```python
from build123d import *

# Parameters (mm, degrees)
SKETCH_W     = 210
SKETCH_H     = 82
SKETCH_R     = 1.65
PAD_DEPTH    = 1.5
POCKET_DEPTH = 1.501


with BuildPart() as part:
    # Sketch → Pad (new body)
    with BuildSketch(Plane.XZ):
        Rectangle(SKETCH_W, SKETCH_H)
        with Locations((100, 30)):
            Circle(SKETCH_R, mode=Mode.SUBTRACT)
        with Locations((100, 10)):
            Circle(SKETCH_R, mode=Mode.SUBTRACT)
        with Locations((100, -30)):
            Circle(SKETCH_R, mode=Mode.SUBTRACT)
        with Locations((100, -10)):
            Circle(SKETCH_R, mode=Mode.SUBTRACT)
        with Locations((-100, 30)):
            Circle(SKETCH_R, mode=Mode.SUBTRACT)
        with Locations((-100, 10)):
            Circle(SKETCH_R, mode=Mode.SUBTRACT)
        with Locations((-100, -30)):
            Circle(SKETCH_R, mode=Mode.SUBTRACT)
        with Locations((-100, -10)):
            Circle(SKETCH_R, mode=Mode.SUBTRACT)
    extrude(amount=PAD_DEPTH)

    # Sketch002 → Pocket (cut, through all)
    with BuildSketch(Plane.XZ.offset(1.5)):
        with BuildLine():
            ThreePointArc((-82.5, 12.5), (-95, 0), (-82.5, -12.5))
            Line((-82.5, -12.5), (82.5, -12.5))
            ThreePointArc((82.5, -12.5), (95, 0), (82.5, 12.5))
            Line((-82.5, 12.5), (82.5, 12.5))
        make_face()
    extrude(amount=-POCKET_DEPTH, mode=Mode.SUBTRACT)


solid = part.part
```
The model under review builds one solid part; all positions refer to its coordinate system, in mm. Coordinates: 2 decimals unless noted, no trailing zeros. Order: outer loops, then holes, each group sorted by start corner. A loop starts at its lowest first (then second) coordinate and runs counter-clockwise, first axis right, second up. Notation, with made-up numbers: M 67,38 L 124,38 A17 ccw 124,46 Z; hole C 82,22.5 d11. An arc over 180 degrees is marked long. One line per question, with ' | ' between items.
(1) The part is to be moulded in two halves that separate along X. For faces 1 (the face through (95, -1, 0)), 2 (the face through (-1, 0, 19)), 3 (the face through (-95, -1, 0)), say which applies: +X half, -X half, draft (parallel to the pull), parting line (faces both ways), or undercut.
Geometry results:
face 1: undercut | face 2: draft | face 3: undercut
(2) Add section C-C, the plane y = -1.15. State how many separate pieces and enclosed holes the cut face has, then the cut area to 3 significant figures.
Geometry results:
separate pieces: 1 | enclosed holes: 9 | area: 12,500 mm²
(3) Add section B-B, the plane z = 5. Write out the cut boundary in (x, y).
Geometry results:
outline: M -105,-1.5 L -93.96,-1.5 L -93.96,0 L -105,0 Z; M 93.96,-1.5 L 105,-1.5 L 105,0 L 93.96,0 Z
(4) Add section A-A, the plane x = -80. Write out the cut boundary in (y, z).
Geometry results:
outline: M -1.5,-41 L 0,-41 L 0,-12.5 L -1.5,-12.5 Z; M -1.5,12.5 L 0,12.5 L 0,41 L -1.5,41 Z
(5) For probe 1 along Z at (x, y) = (100, -0.45); probe 2 along Z at (x, y) = (-79, -0.1); probe 3 along X at (y, z) = (-0.3, 31), list the stretches that pass through material, from the lowest coordinate up. Write a range as from..to.
Geometry results:
probe 1: z = -41..-31.65, -28.35..-11.65, -8.35..8.35, 11.65..28.35, 31.65..41 | probe 2: z = -41..-12.5, 12.5..41 | probe 3: x = -105..-101.31, -98.69..98.69, 101.31..105
(6) Insertion check: pin 1 (3 mm diameter, centred on x = -100, z = 30, fed in from +Y). The pin has a flat end and moves straight along its axis. Give the tip position at first contact, or say it passes through.
Geometry results:
pin 1: passes through
